Build history of the part. All positions in model axes, mm. A direction names the side the tool comes from. Give positions to 0.01 mm unless a question says otherwise; leave off trailing zeros. Order: outer loops, then holes, each group sorted by start corner. A loop starts at its lowest first (then second) coordinate and runs counter-clockwise, first axis right, second up. Notation, with made-up numbers: (37, 47.5) - (56, 47.5) arc R19 ccw to (56, 68.5) - close; hole circle Ø9 at (54.5, 89). An arc over 180 degrees is marked (long way). Use a Markdown table: item, result.
from build123d import *

# Parameters (mm, degrees)
PAD_DEPTH    = 10
SKETCH001_R  = 1.6
POCKET_DEPTH = 5
FILLET_R     = 4
FILLET001_R  = 1


with BuildPart() as part:
    # Sketch → Pad (new body)
    with BuildSketch(Plane.XZ):
        Polygon((0, 0), (0, 5), (8, 5), (8, 20), (9, 20), (9, 10), (24, 10), (24, 8), (9, 8), (9, 0), align=None)
    extrude(amount=PAD_DEPTH)

    # Sketch001 (on Face2 of Pad) → Pocket (cut)
    with BuildSketch(Plane(origin=(0, 0, 5), x_dir=(-1, 0, 0), z_dir=(0, 0, 1))):
        with Locations((-5, 5)):
            Circle(SKETCH001_R)
    extrude(amount=-POCKET_DEPTH, mode=Mode.SUBTRACT)

    # Fillet
    fillet_edges = [part.edges().sort_by_distance(p)[0] for p in [
        (0, 0, 2.5),
        (0, -10, 2.5),
    ]]
    fillet(fillet_edges, radius=FILLET_R)

    # Fillet001
    fillet001_edges = [part.edges().sort_by_distance(p)[0] for p in [
        (8, -5, 5),
    ]]
    fillet(fillet001_edges, radius=FILLET001_R)


solid = part.part
1) Tool access for faces 4 (the flat face through (3, -5, 5)), 5 (the flat face through (16, -5, 10)), 6 (the flat face through (9, -5, 4)), 7 (the flat face through (11, -10, 9)): list every direction of +Z, -Z, +X, -X, +Y, -Y with a clear straight run to the whole face (end or side of a thin tool).
Computed:
| item | result |
|---|---|
| face 4 | +Z, -X, +Y, -Y |
| face 5 | +Z, +X, +Y, -Y |
| face 6 | -Z, +X, +Y, -Y |
| face 7 | +Z, -Z, +X, -X, -Y |
2) Slice it at B-B (x = 5). Write the cut outline in (y, z), and give its area (3 significant figures).
Computed:
| item | result |
|---|---|
| outline | (-10, 0) - (-6.6, 0) - (-6.6, 5) - (-10, 5) - close; (-3.4, 0) - (0, 0) - (0, 5) - (-3.4, 5) - close |
| area | 34.0 mm² |
3) Slice it at C-C (y = -1). Write the cut outline in (x, z), and give its area (3 significant figures).
Computed:
| item | result |
|---|---|
| outline | (1.35, 0) - (9, 0) - (9, 8) - (24, 8) - (24, 10) - (9, 10) - (9, 20) - (8, 20) - (8, 6) arc R1 cw to (7, 5) - (1.35, 5) - close |
| area | 83.4 mm² |
4) Slice it at A-A (y = -5). Write the cut outline in (x, z).
Computed:
| item | result |
|---|---|
| outline | (0, 0) - (3.4, 0) - (3.4, 5) - (0, 5) - close; (6.6, 0) - (9, 0) - (9, 8) - (24, 8) - (24, 10) - (9, 10) - (9, 20) - (8, 20) - (8, 6) arc R1 cw to (7, 5) - (6.6, 5) - close |
5) Pin check, flat tips, straight feed: P1, Ø2.5, axis at y = -7, z = 4.5, coming from the +X side; P2, Ø2, axis at x = 10.5, y = -9, coming from the +Z side; P3, Ø6, axis at x = 18, y = -8.5, coming from the -Z side. Stop position of each tip, or through.
Computed:
| item | result |
|---|---|
| P1 | stops at x = 9 |
| P2 | stops at z = 10 |
| P3 | stops at z = 8 |
6) Wall check: line 1 (Y direction, x = 5, z = 3.05); line 2 (X direction, y = -5, z = 2.65); line 3 (Z direction, x = 14, y = -3.75). Give the ranges that are in metal, low to high. Write a range as from..to.
Computed:
| item | result |
|---|---|
| line 1 | y = -10..-6.6, -3.4..0 |
| line 2 | x = 0..3.4, 6.6..9 |
| line 3 | z = 8..10 |
7) Two-plate mould, pull along Y, no slides. Class faces 1 (the cylindrical face through (6.27, -4.03, 2.54)), 2 (the cylindrical face through (1.141, -8.797, 2.535)), 3 (the flat face through (9, -5, 15)): +Y half, -Y half, draft (parallel to the pull), parting line (faces both ways), or undercut.
Computed:
| item | result |
|---|---|
| face 1 | undercut |
| face 2 | -Y half |
| face 3 | draft |
8) Slice it at D-D (z = 17). Write the cut outline in (x, y), and give its area (3 significant figures).
Computed:
| item | result |
|---|---|
| outline | (8, -10) - (9, -10) - (9, 0) - (8, 0) - close |
| area | 10.0 mm² |
